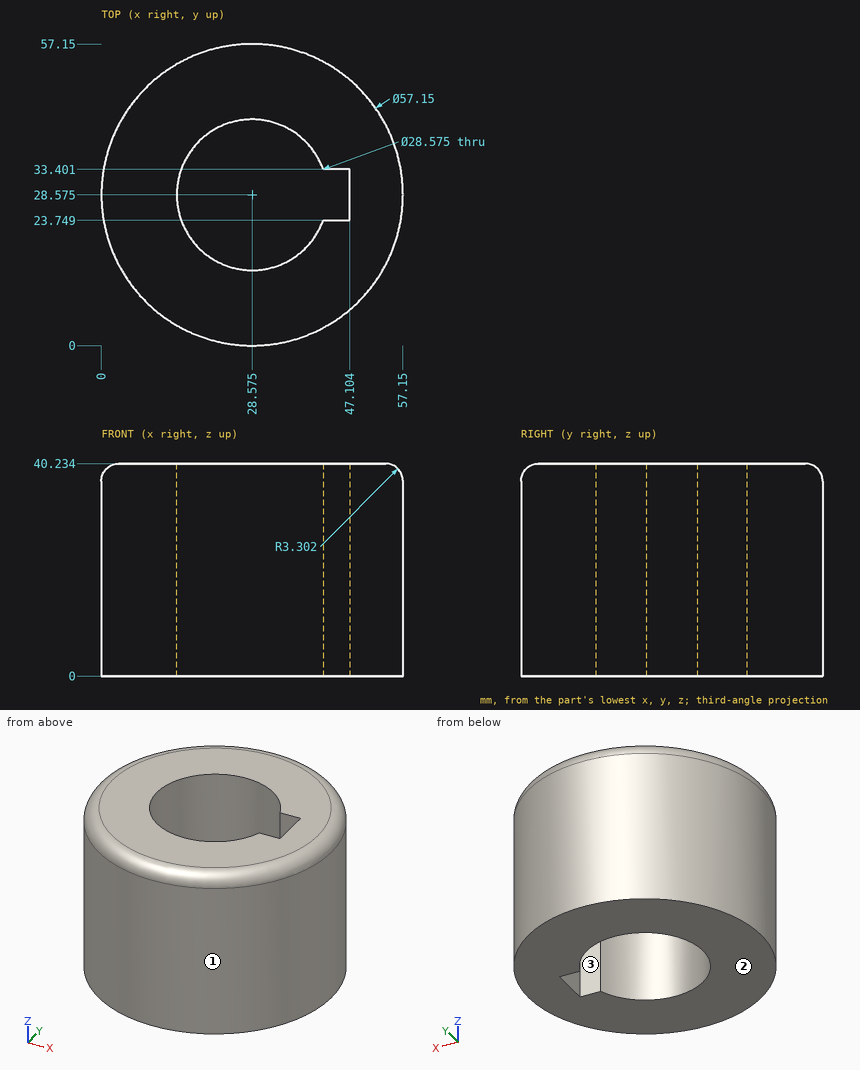
Here's the drawing with two shaded views (mm, measured from the low corner). I have some questions. Coordinates: 2 decimals unless noted, no trailing zeros. Use a Markdown table: item, result. Add a question column.
(1) We'd pull the mould along Y, two halves only. Please class the marked faces 1, 2 and 3: +Y half, -Y half, draft (parallel to the pull), parting line (faces both ways), or undercut.
(2) I'm going to push flat-ended pins straight in: P1, Ø8, axis at y = 48.5, z = 33, coming from the +X side; P2, Ø4, axis at y = 8.5, z = 21.5, coming from the -X side; P3, Ø2, axis at x = 26.5, z = 26, coming from the -Y side. Where does each tip first touch, or does it pass through?
(3) Please list where these lines run through material, in increasing order: line 1 (X direction, y = 28, z = 35) (1 decimal); line 2 (Y direction, x = 16, z = 15.5) (1 decimal); line 3 (Y direction, x = 19.5, z = 14).
Outcome:
| question | item | result |
|---|---|---|
| 1 | face 1 | parting line |
| 1 | face 2 | draft |
| 1 | face 3 | undercut |
| 2 | P1 | stops at x = 52.3 |
| 2 | P2 | stops at x = 6.44 |
| 2 | P3 | stops at y = 0.02 |
| 3 | line 1 | x = 0 to 14.3, 47.1 to 57.1 |
| 3 | line 2 | y = 2.9 to 21.8, 35.4 to 54.2 |
| 3 | line 3 | y = 1.48 to 17.54, 39.61 to 55.67 |
